```python
from build123d import *

# Parameters (mm, degrees)
EXTRUDE_1_DEPTH     = 5.25
CUT_EXTRUDE_1_REACH = 19.808
SKETCH_2_R          = 1.5
SKETCH_2_R_2        = 1


with BuildPart() as part:
    # 草图1 → 凸台-拉伸1 (new body)
    with BuildSketch(Plane(origin=(0, 0, 0), x_dir=(1, 0, 0), z_dir=(0, 1, 0))):
        with BuildLine():
            Line((0, 3), (13.75, 3))
            ThreePointArc((13.75, 3), (16.75, 0), (13.75, -3))
            Line((13.75, -3), (0, -3))
            ThreePointArc((0, -3), (-3, 0), (0, 3))
        make_face()
    extrude(amount=EXTRUDE_1_DEPTH)

    # 草图2 → 切除-拉伸1 (cut, up to next)
    with BuildSketch(Plane(origin=(0, 5.25, 0), x_dir=(1, 0, 0), z_dir=(0, 1, 0)), mode=Mode.PRIVATE) as cut_extrude_1_sk1:
        with Locations(Location((0, 0, 0), (0, 0, 270))):
            Circle(SKETCH_2_R)
    cut_extrude_1_tool1 = extrude(cut_extrude_1_sk1.sketch, amount=-CUT_EXTRUDE_1_REACH, mode=Mode.PRIVATE) & part.part
    # 草图2 → 切除-拉伸1 (cut, up to next)
    with BuildSketch(Plane(origin=(0, 5.25, 0), x_dir=(1, 0, 0), z_dir=(0, 1, 0)), mode=Mode.PRIVATE) as cut_extrude_1_sk2:
        with Locations(Location((13.75, 0, 0), (0, 0, 270))):
            Circle(SKETCH_2_R_2)
    cut_extrude_1_tool2 = extrude(cut_extrude_1_sk2.sketch, amount=-CUT_EXTRUDE_1_REACH, mode=Mode.PRIVATE) & part.part
    add(cut_extrude_1_tool1.solids().sort_by_distance((0, 5.25, 0))[0], mode=Mode.SUBTRACT)
    add(cut_extrude_1_tool2.solids().sort_by_distance((13.75, 5.25, 0))[0], mode=Mode.SUBTRACT)


solid = part.part
```
Could you check a few things on this model? Use its own coordinates, in mm. Round coordinates to 2 decimals unless told otherwise and drop trailing zeros. Loops run counter-clockwise (first coordinate to the right, second up) from the corner with the lowest first, then second, coordinate; pieces in that order, holes last. Notation, with made-up numbers: (87.5, 11) - (145.5, 11) arc R15 cw to (145.5, 26) - close; hole circle Ø9 at (-11.5, 43.25). An arc over 180 degrees is marked (long way). Use CSV: the item, a comma, the result in double quotes.
Item 1: If we section it at D-D on z = 1.25: List the corners of the cut face in (x, y) for me.
Here are the results:
outline,"(-2.73, 0) - (-0.83, 0) - (-0.83, 5.25) - (-2.73, 5.25) - close; (0.83, 0) - (16.48, 0) - (16.48, 5.25) - (0.83, 5.25) - close"
Item 2: If we section it at B-B on x = 14: List the corners of the cut face in (y, z) for me.
Here are the results:
outline,"(0, -2.99) - (5.25, -2.99) - (5.25, -0.97) - (0, -0.97) - close; (0, 0.97) - (5.25, 0.97) - (5.25, 2.99) - (0, 2.99) - close"
Item 3: I need wall thicknesses on L1, parallel to X at y = 1.9, z = 0; L2, parallel to X at y = 3.9, z = -1.35; L3, parallel to X at y = 4.55, z = -2.05. Which ranges of each line are inside material? Lowest first, please. Write a range as [from, to].
Here are the results:
L1,"x = [-3, -1.5], [1.5, 12.75], [14.75, 16.75]"
L2,"x = [-2.68, -0.65], [0.65, 16.43]"
L3,"x = [-2.19, 15.94]"
Item 4: Will these pins go through, and if not, where does the flat tip stop? pin 1 (2 mm diameter, centred on y = 2, z = 1, fed in from -X); pin 2 (1.5 mm diameter, centred on y = 0.5, z = -2, fed in from +X); pin 3 (1 mm diameter, centred on y = 4, z = 1.5, fed in from -X); pin 4 (1.5 mm diameter, centred on y = 1.5, z = -1, fed in from +X).
Here are the results:
pin 1,"stops at x = -3"
pin 2,"stops at x = 16.48"
pin 3,"stops at x = -2.83"
pin 4,"stops at x = 16.74"
Item 5: If we section it at A-A on z = 0: List the corners of the cut face in (x, y) for me.
Here are the results:
outline,"(-3, 0) - (-1.5, 0) - (-1.5, 5.25) - (-3, 5.25) - close; (1.5, 0) - (12.75, 0) - (12.75, 5.25) - (1.5, 5.25) - close; (14.75, 0) - (16.75, 0) - (16.75, 5.25) - (14.75, 5.25) - close"
Item 6: If we section it at C-C on y = 0.7: List the corners of the cut face in (x, z) for me, then the cut area to 3 significant figures.
Here are the results:
outline,"(0, -3) - (13.75, -3) arc R3 ccw to (13.75, 3) - (0, 3) arc R3 ccw to start; hole circle Ø3 at (0, 0); hole circle Ø2 at (13.75, 0)"
area,"101 mm²"
